Check sheet for the modelled part. Datum: model origin and axes. Units: mm. A direction names the side the tool comes from. Give positions to 0.01 mm unless a question says otherwise; leave off trailing zeros. Write each loop counter-clockwise with the first axis right and the second up, starting at its lowest first coordinate (ties: lowest second). Pieces come first, ordered by that corner, then holes.
from build123d import *

# Parameters (mm, degrees)
F0_R     = 4.7625
F1_DEPTH = 9.525


with BuildPart() as f1:
    # F0 (on Top) → F1 (new body)
    with BuildSketch(Plane.XY):
        with BuildLine():
            ThreePointArc((0, 6.35), (1.859872, 1.859872), (6.35, 0))
            Line((6.35, 0), (31.75, 0))
            ThreePointArc((31.75, 0), (36.240128, 1.859872), (38.1, 6.35))
            Line((38.1, 6.35), (38.1, 47.606992))
            ThreePointArc((38.1, 47.606992), (38.776838, 50.459662), (40.663064, 52.704208))
            Line((40.663064, 52.704208), (71.762101, 75.17053))
            ThreePointArc((71.762101, 75.17053), (72.2884, 76.2), (71.762101, 77.22947))
            Line((71.762101, 77.22947), (40.663064, 99.695792))
            ThreePointArc((40.663064, 99.695792), (38.776838, 101.940338), (38.1, 104.793008))
            Line((38.1, 104.793008), (38.1, 146.05))
            ThreePointArc((38.1, 146.05), (36.240128, 150.540128), (31.75, 152.4))
            Line((31.75, 152.4), (6.35, 152.4))
            ThreePointArc((6.35, 152.4), (1.859872, 150.540128), (0, 146.05))
            Line((0, 146.05), (0, 6.35))
        make_face()
        with Locations((19.05, 19.05)):
            Circle(F0_R, mode=Mode.SUBTRACT)
        with Locations((19.05, 133.35)):
            Circle(F0_R, mode=Mode.SUBTRACT)
    extrude(amount=F1_DEPTH)


solid = f1.part
1) Sectioned sample at D-D on y = 125. Record the boundary of the cut face in (x, z) (3 decimals), then the cut area to 3 significant figures.
2) Sectioned sample at B-B on x = 19.05. Record the boundary of the cut face in (y, z) (1 decimal), then the cut area to 3 significant figures.
3) Sectioned sample at A-A on y = 19.05. Record the boundary of the cut face in (x, z) (1 decimal), then the cut area to 3 significant figures.
4) Scan lines: L1, parallel to Y at x = 19.05, z = 6; L2, parallel to Y at x = 20.5, z = 6; L3, parallel to X at y = 39, z = 3. Record each from-to range of solid material in increasing order.
5) Draft check along Y on faces 4 (the flat face through (0, 77, 5)), 5 (the flat face through (55.995, 63.78, 4.696)), 6 (the cylindrical face through (18.02, 128.7, 4.7)). Enter one of: +Y half, -Y half, draft (parallel to the pull), parting line (faces both ways), or undercut.
6) Gauge pin test, flat ends, axial feed: pin 1 (7.5 mm diameter, centred on x = 19.05, y = 133.35, fed in from +Z); pin 2 (4 mm diameter, centred on x = 36.5, y = 34.5, fed in from -Z). Record the tip position at first contact, or that the pin passes through.
7) Sectioned sample at C-C on z = 3.25. Give the number of separate pieces and of enclosed holes in the cut face, then the cut area to 3 significant figures.
8) Access from +Z, -Z, +X, -X, +Y, -Y to the whole of each face (thin tool, end or side, straight path). Record for faces 1 (the flat face through (38.1, 125, 5)), 2 (the flat face through (20, 77, 0)), 3 (the flat face through (38.1, 27, 5)).
Answers below:
1. outline: (0, 0) - (38.1, 0) - (38.1, 9.525) - (0, 9.525) - close
1. area: 363 mm2
2. outline: (0, 0) - (14.3, 0) - (14.3, 9.5) - (0, 9.5) - close; (23.8, 0) - (128.6, 0) - (128.6, 9.5) - (23.8, 9.5) - close; (138.1, 0) - (152.4, 0) - (152.4, 9.5) - (138.1, 9.5) - close
2. area: 1,270 mm2
3. outline: (0, 0) - (14.3, 0) - (14.3, 9.5) - (0, 9.5) - close; (23.8, 0) - (38.1, 0) - (38.1, 9.5) - (23.8, 9.5) - close
3. area: 272 mm2
4. L1: y = 0 to 14.29, 23.81 to 128.59, 138.11 to 152.4
4. L2: y = 0 to 14.51, 23.59 to 128.81, 137.89 to 152.4
4. L3: x = 0 to 38.1
5. face 4: draft
5. face 5: -Y half
5. face 6: undercut
6. pin 1: passes through
6. pin 2: stops at z = 0
7. separate pieces: 1
7. enclosed holes: 2
7. area: 6,520 mm2
8. face 1: +Z, -Z, +X, +Y
8. face 2: -Z, +X, -X, +Y, -Y
8. face 3: +Z, -Z, +X, -Y
